Read the model definition and answer for the solid it produces. Units are mm, in the model's axes. Coordinates: 2 decimals unless noted, no trailing zeros. Order: outer loops, then holes, each group sorted by start corner. A loop starts at its lowest first (then second) coordinate and runs counter-clockwise, first axis right, second up. Notation, with made-up numbers: (-24, 86.5) -> (31, 86.5) arc R21 ccw to (31, 107.5) -> close; hole circle Ø10 at (8, 41). An arc over 180 degrees is marked (long way). Answer as a JSON object with one key per item and string values. Group by question number.
1) Section C-C on x = 17.5 is taken. Determine the outline of the cut face in (y, z).
2) Section D-D on z = 1.1 is taken. Count the separate pieces of the cut face and the enclosed holes in it, and give its area (3 significant figures).
3) Section A-A on y = 25 is taken. Determine the outline of the cut face in (x, z).
4) Consider L1, parallel to Y at x = 5, z = 0.8; L2, parallel to Y at x = 30, z = 1.2; L3, parallel to X at y = 10, z = 0.2. Determine where each line is inside the solid, lowest interval first.
5) Section B-B on y = -13 is taken. Determine the outline of the cut face in (x, z), and give its area (3 significant figures).
from build123d import *

# Parameters (mm, degrees)
SKETCH1_R           = 6.5
SKETCH1_R_2         = 1.5
SKETCH1_R_3         = 3
BOSS_EXTRUDE1_DEPTH = 1.5875
FILLET1_R           = 5
FILLET2_R           = 13


with BuildPart() as part:
    # Sketch1 → Boss-Extrude1 (new body)
    with BuildSketch(Plane.XY):
        Polygon((0, 0), (0, 50), (35, 50), (35, 0), (106.009911505, -84.626317146), (72.668567607, -112.603026514), (0, -26), align=None)
        with Locations((17.5, -13)):
            Circle(SKETCH1_R, mode=Mode.SUBTRACT)
        with Locations((5, 45)):
            Circle(SKETCH1_R_2, mode=Mode.SUBTRACT)
        with Locations((5, 25)):
            Circle(SKETCH1_R_2, mode=Mode.SUBTRACT)
        with Locations((5, 5)):
            Circle(SKETCH1_R_2, mode=Mode.SUBTRACT)
        with Locations(Location((30, 5, 0), (0, 0, 180))):
            Circle(SKETCH1_R_2, mode=Mode.SUBTRACT)
        with Locations(Location((30, 25, 0), (0, 0, 180))):
            Circle(SKETCH1_R_2, mode=Mode.SUBTRACT)
        with Locations(Location((30, 45, 0), (0, 0, 180))):
            Circle(SKETCH1_R_2, mode=Mode.SUBTRACT)
        with Locations((75.350884872, -81.943999881)):
            Circle(SKETCH1_R_3, mode=Mode.SUBTRACT)
        with Locations((53.004955752, -55.313158573)):
            Circle(SKETCH1_R_2, mode=Mode.SUBTRACT)
    extrude(amount=BOSS_EXTRUDE1_DEPTH)

    # Fillet1
    fillet1_edges = [part.edges().sort_by_distance(p)[0] for p in [
        (0, 50, 0.79375),
        (35, 50, 0.79375),
    ]]
    fillet(fillet1_edges, radius=FILLET1_R)

    # Fillet2
    fillet2_edges = [part.edges().sort_by_distance(p)[0] for p in [
        (35, 0, 0.79375),
        (106.009911505, -84.626317146, 0.79375),
        (72.668567607, -112.603026514, 0.79375),
        (0, -26, 0.79375),
    ]]
    fillet(fillet2_edges, radius=FILLET2_R)


solid = part.part
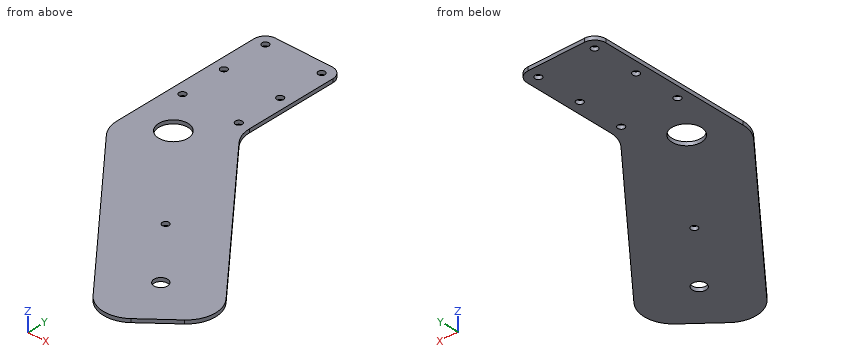
Worked answers:
{
 "1": {"outline": "(-46.86, 0) -> (-19.5, 0) -> (-19.5, 1.59) -> (-46.86, 1.59) -> close; (-6.5, 0) -> (50, 0) -> (50, 1.59) -> (-6.5, 1.59) -> close"},
 "2": {"separate pieces": "1", "enclosed holes": "9", "area": "6,780 mm²"},
 "3": {"outline": "(0, 0) -> (3.5, 0) -> (3.5, 1.59) -> (0, 1.59) -> close; (6.5, 0) -> (28.5, 0) -> (28.5, 1.59) -> (6.5, 1.59) -> close; (31.5, 0) -> (35, 0) -> (35, 1.59) -> (31.5, 1.59) -> close"},
 "4": {"L1": "y = -31.96 to 3.5, 6.5 to 23.5, 26.5 to 43.5, 46.5 to 50", "L2": "y = -61.75 to 3.5, 6.5 to 23.5, 26.5 to 43.5, 46.5 to 50", "L3": "x = 0 to 35"},
 "5": {"outline": "(0, 0) -> (11, 0) -> (11, 1.59) -> (0, 1.59) -> close; (24, 0) -> (45.91, 0) -> (45.91, 1.59) -> (24, 1.59) -> close", "area": "52.2 mm²"}
}
